Verification items for the finished model (mm, model axes). Face numbers are marked on the shaded views. A direction names the side the tool comes from. Round coordinates to 2 decimals unless told otherwise and drop trailing zeros. Write each loop counter-clockwise with the first axis right and the second up, starting at its lowest first coordinate (ties: lowest second). Pieces come first, ordered by that corner, then holes. Notation, with made-up numbers: M 23.25,6.25 L 45.25,6.25 A23 ccw 45.25,19.25 Z; hole C -27,-34 d1. An arc over 180 degrees is marked long. Answer in a Markdown table with one row per item. Add a question column.
1. Material ranges on probe 1 along Y at (x, z) = (-18, 2.3); probe 2 along Z at (x, y) = (19.5, -13); probe 3 along X at (y, z) = (10, 8.5), recorded low to high.
2. Go/stop test with flat-tipped pins: pin 1 Ø3 at (x, z) = (9.5, 10) entering from +Y; pin 2 Ø4 at (x, y) = (18, -18.5) entering from +Z; pin 3 Ø1.1 at (x, y) = (12, -1.5) entering from -Z; pin 4 Ø13 at (x, y) = (13, 3.5) entering from +Z. Record where each tip stops, or that it passes through.
3. Sectioned sample at B-B on x = -2. Record the cut outline in (y, z), plus the area to 3 significant figures.
4. Draft check along Y on the marked faces 5, 6, 7 and 8. Enter one of: pulls with the +Y half, pulls with the -Y half, needs draft (parallel to the pull), parting line crosses it, or undercut.
5. Sectioned sample at A-A on x = 18. Record the cut outline in (y, z).
6. Set-up check for the marked faces 1, 2, 3 and 4: record each of +Z, -Z, +X, -X, +Y, -Y from which the full face is reachable in a straight line by a thin tool's end or side.
7. Sectioned sample at C-C on y = -18.5. Record the cut outline in (x, z).
8. Sectioned sample at D-D on x = -17.5. Record the cut outline in (y, z).
```python
from build123d import *

# Parameters (mm, degrees)
SKETCH1_W                           = 44
SKETCH1_H                           = 45
BASE_DEPTH                          = 5
WIRE_GROOVES_DEPTH                  = 51.338851795
SLANTED_START                       = -22
SLANTED_SCREW_PLATFORM_DEPTH        = 9
MOUNTING_HOLE_SCREW_INSERTION_DEPTH = 36.040152348
SKETCH6_W                           = 5
SKETCH6_H                           = 3
ZIP_TIE_SLOTS_DEPTH                 = 34.699235283
SKETCH7_R                           = 1.75
MOUNT_CLAMPING_HOLES_DEPTH          = 34.699235283
EDGE_FILLETS_R                      = 1


with BuildPart() as part:
    # Sketch1 → Base (new body)
    with BuildSketch(Plane.XY):
        Rectangle(SKETCH1_W, SKETCH1_H)
    extrude(amount=BASE_DEPTH)

    # Sketch2 → Wire Grooves (cut, through all)
    with BuildSketch(Plane(origin=(0, 22.5, 0), x_dir=(1, 0, 0), z_dir=(0, 1, 0))):
        with BuildLine():
            Line((-14.9, 0), (-8.9, 0))
            ThreePointArc((-8.9, 0), (-9.456497116, -1.343502884), (-10.8, -1.9))
            Line((-10.8, -1.9), (-13, -1.9))
            ThreePointArc((-13, -1.9), (-14.343502884, -1.343502884), (-14.9, 0))
        make_face()
        with BuildLine():
            Line((13, -1.9), (10.8, -1.9))
            ThreePointArc((10.8, -1.9), (9.456497116, -1.343502884), (8.9, 0))
            Line((8.9, 0), (14.9, 0))
            ThreePointArc((14.9, 0), (14.343502884, -1.343502884), (13, -1.9))
        make_face()
    extrude(amount=-WIRE_GROOVES_DEPTH, mode=Mode.SUBTRACT)

    # Sketch4 → Slanted Screw Platform (add, symmetric)
    with BuildSketch(Plane(origin=(22, 0, 0), x_dir=(0, 0, -1), z_dir=(1, 0, 0)).offset(SLANTED_START)):
        Polygon((-5, -22.5), (-5, 22.5), (-17.057713659, 22.5), align=None)
    extrude(amount=SLANTED_SCREW_PLATFORM_DEPTH, both=True)

    # Sketch5 → Mounting Hole Screw Insertion (cut, through all)
    with BuildSketch(Plane(origin=(0, -2.757214207, 10.290063509), x_dir=(1, 0, 0), z_dir=(0, -0.2588190451025216, 0.9659258262890681))):
        with BuildLine():
            Line((-4, 19.25), (4, 19.25))
            ThreePointArc((4, 19.25), (6.75, 16.5), (4, 13.75))
            Line((4, 13.75), (-4, 13.75))
            ThreePointArc((-4, 13.75), (-6.75, 16.5), (-4, 19.25))
        make_face()
    extrude(amount=-MOUNTING_HOLE_SCREW_INSERTION_DEPTH, mode=Mode.SUBTRACT)

    # Sketch6 → Zip Tie Slots (cut, through all)
    with BuildSketch(Plane.XY.offset(5)):
        with Locations((-17.9, 18)):
            Rectangle(SKETCH6_W, SKETCH6_H)
        with Locations((17.9, 18)):
            Rectangle(SKETCH6_W, SKETCH6_H)
    extrude(amount=-ZIP_TIE_SLOTS_DEPTH, mode=Mode.SUBTRACT)

    # Sketch7 → Mount Clamping Holes (cut, through all)
    with BuildSketch(Plane.XY.offset(5)):
        with Locations((-18, -18.5)):
            Circle(SKETCH7_R)
        with Locations(Location((18, -18.5, 0), (0, 0, 180))):
            Circle(SKETCH7_R)
    extrude(amount=-MOUNT_CLAMPING_HOLES_DEPTH, mode=Mode.SUBTRACT)

    # Edge Fillets
    edge_fillets_edges = [part.edges().sort_by_distance(p)[0] for p in [
        (-22, 0, 5),
        (-15.5, 22.5, 5),
        (-9, 22.5, 11.02885683),
        (0, 22.5, 17.057713659),
        (22, 0, 5),
        (9, 22.5, 11.02885683),
        (22, -22.5, 2.5),
        (-22, -22.5, 2.5),
        (-22, 22.5, 2.5),
        (22, 22.5, 2.5),
        (15.5, 22.5, 5),
    ]]
    fillet(edge_fillets_edges, radius=EDGE_FILLETS_R)


solid = part.part
```
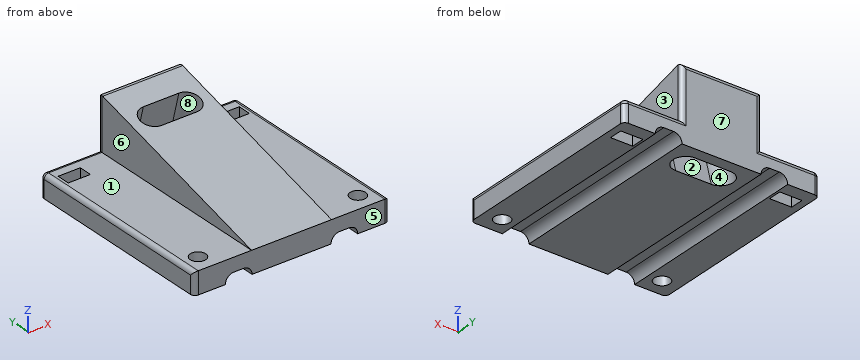
Geometry check:
| question | item | result |
|---|---|---|
| 1 | probe 1 | y = -22.5 to -20.25, -16.75 to 16.5, 19.5 to 22.5 |
| 1 | probe 2 | z = 0 to 5 |
| 1 | probe 3 | x = -9 to 9 |
| 2 | pin 1 | stops at y = 22.5 |
| 2 | pin 2 | stops at z = 5 |
| 2 | pin 3 | stops at z = 1.9 |
| 2 | pin 4 | stops at z = 13.34 |
| 3 | outline | M -22.5,0 L 14.24,0 L 10.52,13.85 L -22.5,5 Z; M 15.84,15.27 L 19.93,0 L 22.5,0 L 22.5,15.75 A1 ccw 21.24,16.72 Z |
| 3 | area | 413 mm2 |
| 4 | face 5 | pulls with the -Y half |
| 4 | face 6 | needs draft |
| 4 | face 7 | pulls with the +Y half |
| 4 | face 8 | undercut |
| 5 | outline | M -22.5,0 L -20.25,0 L -20.25,5 L -22.5,5 Z; M -16.75,0 L 16.5,0 L 16.5,5 L -16.75,5 Z; M 19.5,0 L 22.5,0 L 22.5,4 A1 ccw 21.5,5 L 19.5,5 Z |
| 6 | face 1 | +Z, -X, +Y, -Y |
| 6 | face 2 | +Z |
| 6 | face 3 | +Z, +X, +Y, -Y |
| 6 | face 4 | none |
| 7 | outline | M -22,0 L -19.75,0 L -19.75,5 L -21,5 A1 ccw -22,4 Z; M -16.25,0 L -14.9,0 A1.9 cw -13,1.9 L -10.8,1.9 A1.9 cw -8.9,0 L 8.9,0 A1.9 cw 10.8,1.9 L 13,1.9 A1.9 cw 14.9,0 L 16.25,0 L 16.25,5 L 9,5 L 9,6.07 L -9,6.07 L -9,5 L -16.25,5 Z; M 19.75,0 L 22,0 L 22,4 A1 ccw 21,5 L 19.75,5 Z |
| 8 | outline | M -22.5,0 L -20.18,0 L -20.18,5 L -22.5,5 Z; M -16.82,0 L 16.5,0 L 16.5,5 L -16.82,5 Z; M 19.5,0 L 22.5,0 L 22.5,4 A1 ccw 21.5,5 L 19.5,5 Z |
